Read the model definition and answer for the solid it produces. Units are mm, in the model's axes. A direction names the side the tool comes from. Coordinates: 2 decimals unless noted, no trailing zeros. Write each loop counter-clockwise with the first axis right and the second up, starting at its lowest first coordinate (ties: lowest second). Pieces come first, ordered by that corner, then holes. Notation, with made-up numbers: (18, 46) -> (40, 46) arc R19 cw to (40, 55) -> close; hole circle Ø7 at (-23.5, 36.25). An arc over 180 degrees is marked (long way). Use CSV: the item, a comma, the result in double quotes.
from build123d import *

# Parameters (mm, degrees)
BASEHEAD_DEPTH     = 6.63
INDENT_START       = -0.82875
INDENT_2_OUTLINE_R = 7
INDENT_2_DEPTH     = 0.82875
SKETCH4_W          = 0.6
SKETCH4_H          = 11.237604307
THDSCHPAT_COUNT    = 16
THDSCHPAT_PITCH    = 1.46875


# Read off the part's stored shape, not the designer's step: Indent
with BuildPart() as part:
    # Sketch1 → BaseHead (new body)
    with BuildSketch(Plane(origin=(0, 0, 0), x_dir=(0, 0, -1), z_dir=(1, 0, 0))):
        Polygon((8, 4.618802154), (8, -4.618802154), (0, -9.237604307), (-8, -4.618802154), (-8, 4.618802154), (0, 9.237604307), align=None)
    extrude(amount=BASEHEAD_DEPTH)

    # Indent outline → Indent (revolve)
    with BuildSketch(Plane.YX):
        Polygon((5, 6.63), (5, 30.802), (4.172, 31.63), (0, 31.63), (0, 6.63), align=None)
    revolve(axis=Axis((0, 0, 0), (1, 0, 0)))

    # Indent 2 outline → Indent 2 (cut)
    with BuildSketch(Plane.ZY.offset(INDENT_START)):
        with Locations((0.033212245, 0.192376607)):
            Circle(INDENT_2_OUTLINE_R)
    extrude(amount=INDENT_2_DEPTH, mode=Mode.SUBTRACT)

    # Sketch3 → HeadChamfer (revolve, cut)
    with BuildSketch(Plane.XY, mode=Mode.PRIVATE) as headchamfer_sk:
        Polygon((0, 8), (3.601282526, 14.237604307), (3.601282526, 19.237604307), (-10, 19.237604307), (-10, 8), align=None)
    revolve(headchamfer_sk.sketch.rotate(Axis((0, 0, 0), (1, 0, 0)), 90), axis=Axis((0, 0, 0), (1, 0, 0)), mode=Mode.SUBTRACT)

    # Sketch4 → BearingFace (revolve, cut)
    with BuildSketch(Plane.XY, mode=Mode.PRIVATE) as bearingface_sk:
        with Locations((6.33, 13.618802154)):
            Rectangle(SKETCH4_W, SKETCH4_H)
    revolve(bearingface_sk.sketch.rotate(Axis((0, 0, 0), (1, 0, 0)), 90), axis=Axis((0, 0, 0), (1, 0, 0)), mode=Mode.SUBTRACT)

    # ThdSchSke → ThreadSchematic (revolve, cut)
    with BuildSketch(Plane.XY):
        Polygon((8.13, -4.172), (7.550228158, -5), (7.550228158, -6.25), (8.709771842, -6.25), (8.709771842, -5), align=None)
    threadschematic = revolve(axis=Axis((-3.175, 0, 0), (1, 0, 0)), mode=Mode.SUBTRACT)

    # ThdSchPat: ThreadSchematic ×16
    with Locations(*[(i * THDSCHPAT_PITCH, 0, 0) for i in range(1, THDSCHPAT_COUNT)]):
        add(threadschematic, mode=Mode.SUBTRACT)


solid = part.part
1. A tool of negligible diameter and unlimited length cuts with its end or side. For faces 4 (the cylindrical face through (25.02, -1.08, -4.88)), 5 (the flat face through (6.03, 4.2, 7.2)), 6 (the flat face through (6.03, -4, -7.2)), 7 (the flat face through (2.973, -6.896, -4.056)), from which of +Z, -Z, +X, -X, +Y, -Y can it reach the whole face along a straight path? Write none if from no direction.
Solutions:
face 4,"+X"
face 5,"+Z, +X, +Y"
face 6,"-Z, +X, -Y"
face 7,"-Z, +X, -X, -Y"
2. Find the intervals of material crossed by line 1 along X through (y, z) = (7.25, 0.5); line 2 along X through (y, z) = (0.5, -0.25); line 3 along Y through (x, z) = (19, -0.25), in increasing order.
Solutions:
line 1,"x = 0 to 6.63"
line 2,"x = 0.83 to 31.63"
line 3,"y = -4.99 to 4.99"
3. For a pull along Z with two mould halves and no side action, classify faces 1 (the flat face through (6.03, 4.2, -7.2)), 2 (the cylindrical face through (14.74, -1.08, -4.88)), 3 (the flat face through (0.829, 0, 0)) as pulls with the +Z half, pulls with the -Z half, needs draft (parallel to the pull), parting line crosses it, or undercut.
Solutions:
face 1,"needs draft"
face 2,"parting line crosses it"
face 3,"undercut"
4. Each of these flat-tipped pins is pushed along its axis until it touches: pin 1 Ø5 at (x, z) = (16, 4.5) entering from +Y; pin 2 Ø6 at (x, z) = (27, -5) entering from -Y; pin 3 Ø2.5 at (y, z) = (-8.5, 1.5) entering from +X. Where does it stop, or does it pass through?
Solutions:
pin 1,"stops at y = 4.58"
pin 2,"stops at y = -4.57"
pin 3,"stops at x = 6.63"
5. A cutting plane is placed at A-A (x = 4). Give the vertices of the cut face in (y, z), and give its area (3 significant figures).
Solutions:
outline,"(-9.24, 0) -> (-4.62, -8) -> (4.62, -8) -> (9.24, 0) -> (4.62, 8) -> (-4.62, 8) -> close"
area,"222 mm^2"
